Geometry check sheet. Reference: the model listing, model coordinates, mm. A direction names the side the tool comes from. Round coordinates to 2 decimals unless told otherwise and drop trailing zeros. Loops run counter-clockwise (first coordinate to the right, second up) from the corner with the lowest first, then second, coordinate; pieces in that order, holes last. Notation, with made-up numbers: (57.25, -12.75) -> (91.25, -12.75) arc R9 cw to (91.25, -4.75) -> close; hole circle Ø11 at (37.25, 28.5). An arc over 180 degrees is marked (long way). Use a Markdown table: item, result. Add a question column.
Q1. Sectioned sample at C-C, the plane y = 2.5. Enter the section's corners in (x, z).
Q2. Sectioned sample at D-D, the plane x = 10. Enter the section's corners in (y, z).
Q3. Sectioned sample at A-A, the plane x = 113. Enter the section's corners in (y, z).
Q4. Release check for a two-part mould opening along X. For faces 1 (the face through (-142.5, 4, 1)), 2 (the face through (-1, 4, 5)), 3 (the face through (-2, 0, -1)) record: released by +X, released by -X, zero draft, split by the parting line, or undercut.
Q5. Sectioned sample at B-B, the plane z = 0. Enter the section's corners in (x, y), then the cut area to 3 significant figures.
Q6. Set-up check for faces 4 (the face through (-1, 4, 10)), 5 (the face through (142.5, 4, 1)): record each of +Z, -Z, +X, -X, +Y, -Y from which the full face is reachable in a straight line by a thin tool's end or side.
Q7. Material ranges on L1, parallel to X at y = 3.75, z = 0; L2, parallel to X at y = 0.5, z = 3; L3, parallel to Z at x = 28, y = 0.75, recorded low to high.
```python
from build123d import *

# Parameters (mm, degrees)
SKETCH1_W               = 285
SKETCH1_H               = 100
BOSS_EXTRUDE1_DEPTH     = 7.5
CUT_EXTRUDE1_DEPTH      = 152.20350525
CUT_EXTRUDE1_DEPTH_BACK = 10
SKETCH2_R               = 22.5
SKETCH2_W               = 150
SKETCH2_H               = 5
FILLET1_R               = 2


with BuildPart() as part:
    # Sketch1 → Boss-Extrude1 (new body)
    with BuildSketch(Plane(origin=(0, 0, 0), x_dir=(1, 0, 0), z_dir=(0, 1, 0))):
        Rectangle(SKETCH1_W, SKETCH1_H)
    extrude(amount=BOSS_EXTRUDE1_DEPTH)

    # Sketch2 → Cut-Extrude1 (cut, two sides: drawn at the far end of the back side and taken through both)
    with BuildSketch(Plane(origin=(0, 7.5, 0), x_dir=(1, 0, 0), z_dir=(0, 1, 0)).offset(-CUT_EXTRUDE1_DEPTH_BACK)):
        with Locations(Location((-113, 0, 0), (0, 0, 90))):
            Circle(SKETCH2_R)
        with Locations(Location((113, 0, 0), (0, 0, 90))):
            Circle(SKETCH2_R)
        with Locations((0, -7.5)):
            Rectangle(SKETCH2_W, SKETCH2_H)
    extrude(amount=CUT_EXTRUDE1_DEPTH + CUT_EXTRUDE1_DEPTH_BACK, mode=Mode.SUBTRACT)

    # Fillet1
    fillet1_edges = [part.edges().sort_by_distance(p)[0] for p in [
        (142.5, 3.75, 50),
        (-142.5, 3.75, 50),
        (-142.5, 3.75, -50),
        (142.5, 3.75, -50),
    ]]
    fillet(fillet1_edges, radius=FILLET1_R)


solid = part.part
```
Values:
| question | item | result |
|---|---|---|
| 1 | outline | (-142.5, -48) arc R2 ccw to (-140.5, -50) -> (140.5, -50) arc R2 ccw to (142.5, -48) -> (142.5, 48) arc R2 ccw to (140.5, 50) -> (-140.5, 50) arc R2 ccw to (-142.5, 48) -> close; hole circle Ø45 at (-113, 0); hole (-75, 5) -> (75, 5) -> (75, 10) -> (-75, 10) -> close; hole circle Ø45 at (113, 0) |
| 2 | outline | (0, -50) -> (7.5, -50) -> (7.5, 5) -> (0, 5) -> close; (0, 10) -> (7.5, 10) -> (7.5, 50) -> (0, 50) -> close |
| 3 | outline | (0, -50) -> (7.5, -50) -> (7.5, -22.5) -> (0, -22.5) -> close; (0, 22.5) -> (7.5, 22.5) -> (7.5, 50) -> (0, 50) -> close |
| 4 | face 1 | released by -X |
| 4 | face 2 | undercut |
| 4 | face 3 | zero draft |
| 5 | outline | (-142.5, 0) -> (-135.5, 0) -> (-135.5, 7.5) -> (-142.5, 7.5) -> close; (-90.5, 0) -> (90.5, 0) -> (90.5, 7.5) -> (-90.5, 7.5) -> close; (135.5, 0) -> (142.5, 0) -> (142.5, 7.5) -> (135.5, 7.5) -> close |
| 5 | area | 1,460 mm^2 |
| 6 | face 4 | +Y, -Y |
| 6 | face 5 | +Z, -Z, +X, +Y, -Y |
| 7 | L1 | -142.5 to -135.5, -90.5 to 90.5, 135.5 to 142.5 |
| 7 | L2 | -142.5 to -135.3, -90.7 to 90.7, 135.3 to 142.5 |
| 7 | L3 | -50 to 5, 10 to 50 |
